Can you work these out from the model? Positions are in its coordinate system, mm. Face numbers are marked on the shaded views. Round coordinates to 2 decimals unless told otherwise and drop trailing zeros. Loops run counter-clockwise (first coordinate to the right, second up) from the corner with the lowest first, then second, coordinate; pieces in that order, holes last. Notation, with made-up numbers: M 16,7 L 42,7 A20 ccw 42,41 Z; hole C 58.5,52 d9. An arc over 180 degrees is marked long. Answer as CSV lines item,"result".
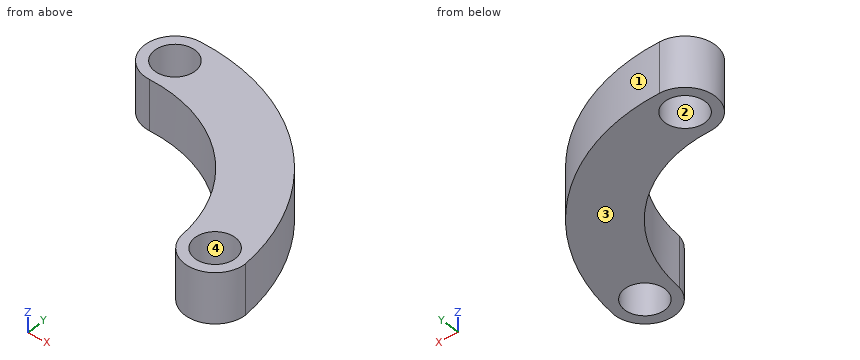
from build123d import *

# Parameters (mm, degrees)
CROQUIS1_R              = 20
SALIENTE_EXTRUIR1_DEPTH = 50


with BuildPart() as part:
    # Croquis1 → Saliente-Extruir1 (new body)
    with BuildSketch(Plane.XY):
        with BuildLine():
            ThreePointArc((140.520313479, -160.563100092), (95.907092551, -67.678686317), (0, -30))
            ThreePointArc((0, -30), (-30, 0), (0, 30))
            ThreePointArc((0, 30), (136.221327258, -23.341808369), (200, -155))
            ThreePointArc((200, -155), (172.793689709, -184.869638394), (140.520313479, -160.563100092))
        make_face()
        with Locations((170, -155)):
            Circle(CROQUIS1_R, mode=Mode.SUBTRACT)
        Circle(CROQUIS1_R, mode=Mode.SUBTRACT)
    extrude(amount=SALIENTE_EXTRUIR1_DEPTH)


solid = part.part
Item 1: If we section it at D-D on x = 35.5: Write out the boundary of the cut face in (y, z).
Output:
outline,"M -34.55,0 L 26.83,0 L 26.83,50 L -34.55,50 Z"
Item 2: Will these pins go through, and if not, where does the flat tip stop? pin 1 (1.5 mm diameter, centred on x = 141.5, z = 40.5, fed in from -Y); pin 2 (8 mm diameter, centred on x = 60, z = 38.5, fed in from -Y).
Output:
pin 1,"stops at y = -166.4"
pin 2,"stops at y = -45.37"
Item 3: If we section it at A-A on z = 8.5: Write out the boundary of the cut face in (x, y).
Output:
outline,"M 0,-30 A140.9 cw 140.52,-160.56 A30 ccw 200,-155 A200.61 ccw 0,30 A30 ccw Z; hole C 0,0 d40; hole C 170,-155 d40"
Item 4: If we section it at B-B on y = 0: Write out the boundary of the cut face in (x, z), then the cut area to 3 significant figures.
Output:
outline,"M -30,0 L -20,0 L -20,50 L -30,50 Z; M 20,0 L 105.53,0 L 105.53,50 L 20,50 Z"
area,"4,780 mm2"
Item 5: If I drill on line 1 along Y through (x, z) = (0, 28); line 2 along Y through (x, z) = (12, 31.5); line 3 along X through (y, z) = (-170, 39.5), over which ranges is the centre line in solid material (lowest first)? Write a range as from..to.
Output:
line 1,"y = -30..-20, 20..30"
line 2,"y = -30.51..-16, 16..29.64"
line 3,"x = 144.02..156.77, 183.23..195.98"
Item 6: If we section it at C-C on x = 170: Write out the boundary of the cut face in (y, z).
Output:
outline,"M -185,0 L -175,0 L -175,50 L -185,50 Z; M -135,0 L -64.1,0 L -64.1,50 L -135,50 Z"
Item 7: We'd pull the mould along Y, two halves only. Please class the marked faces 1, 2, 3 and 4: released by +Y, released by -Y, zero draft, split by the parting line, or undercut.
Output:
face 1,"released by +Y"
face 2,"undercut"
face 3,"zero draft"
face 4,"undercut"
